from build123d import *

# Parameters (mm, degrees)
BOSS_EXTRUDE1_DEPTH = 25
SKETCH2_R           = 2.6
CUT_EXTRUDE1_DEPTH  = 8
CUT_EXTRUDE2_DEPTH  = 25.75
FILLET1_R           = 4
CHAMFER1_SIZE       = 2
CHAMFER2_SIZE       = 1


with BuildPart() as part:
    # Sketch1 → Boss-Extrude1 (new body)
    with BuildSketch(Plane.XY):
        Polygon((0, 14), (0, -14), (7, -14), (7, -5.5), (15, -5.5), (15, -10.75), (24, -10.75), (24, 10.75), (15, 10.75), (15, 5.5), (7, 5.5), (7, 14), align=None)
    extrude(amount=BOSS_EXTRUDE1_DEPTH)

    # Sketch2 → Cut-Extrude1 (cut)
    with BuildSketch(Plane.ZY):
        with Locations(Location((5, 9, 0), (0, 0, 270))):  # turned: the seam where the file's is
            Circle(SKETCH2_R)
        with Locations(Location((20, 9, 0), (0, 0, 270))):  # turned: the seam where the file's is
            Circle(SKETCH2_R)
        with Locations(Location((5, -8, 0), (0, 0, 270))):  # turned: the seam where the file's is
            Circle(SKETCH2_R)
        with Locations(Location((20, -8, 0), (0, 0, 270))):  # turned: the seam where the file's is
            Circle(SKETCH2_R)
    extrude(amount=-CUT_EXTRUDE1_DEPTH, mode=Mode.SUBTRACT)

    # Sketch3 → Cut-Extrude2 (cut, through all)
    with BuildSketch(Plane(origin=(0, 10.75, 0), x_dir=(1, 0, 0), z_dir=(0, 1, 0))):
        Polygon((24, 0), (23.5, -25), (24, -25), align=None)
    extrude(amount=-CUT_EXTRUDE2_DEPTH, mode=Mode.SUBTRACT)

    # Fillet1
    fillet1_edges = [part.edges().sort_by_distance(p)[0] for p in [
        (3.5, -14, 25),
        (3.5, -14, 0),
        (3.5, 14, 0),
        (3.5, 14, 25),
    ]]
    fillet(fillet1_edges, radius=FILLET1_R)

    # Chamfer1
    chamfer1_edges = [part.edges().sort_by_distance(p)[0] for p in [
        (19.25, -10.75, 25),
        (19.25, 10.75, 25),
    ]]
    chamfer(chamfer1_edges, length=CHAMFER1_SIZE)

    # Chamfer2
    chamfer2_edges = [part.edges().sort_by_distance(p)[0] for p in [
        (15, -10.75, 11.5),
        (15, 10.75, 11.5),
        (23.77, -10.75, 11.5),
        (23.77, 10.75, 11.5),
    ]]
    chamfer(chamfer2_edges, length=CHAMFER2_SIZE)


solid = part.part
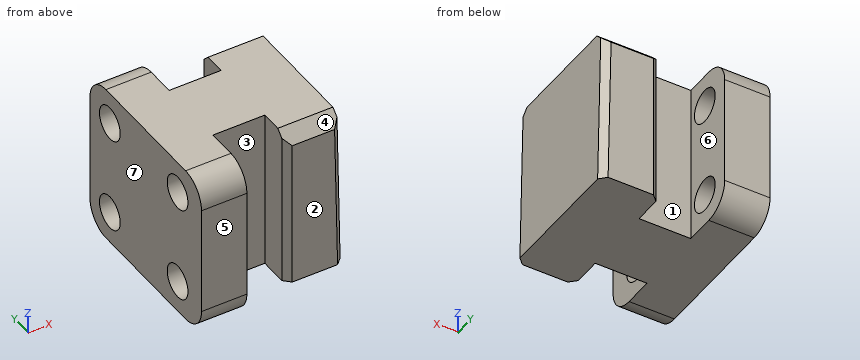
Geometry: final body of the model. Coordinates: model frame, mm. Face numbers are marked on the shaded views. A direction names the side the tool comes from. Coordinates: 2 decimals unless noted, no trailing zeros. Order: outer loops, then holes, each group sorted by start corner. A loop starts at its lowest first (then second) coordinate and runs counter-clockwise, first axis right, second up. Notation, with made-up numbers: (-33.75, -31.75) - (13.25, -31.75) arc R10 cw to (13.25, -13.75) - close; hole circle Ø7 at (86.5, 49). An arc over 180 degrees is marked (long way). Use one line per item in the form item = value.
1) Pin query (flat end, axial travel): pin 1 (7.5 mm diameter, centred on x = 18, z = 8, fed in from -Y); pin 2 (7.5 mm diameter, centred on x = 19, z = 8, fed in from +Y); pin 3 (4 mm diameter, centred on x = 12.5, z = 13, fed in from +Y). Return the tip coordinate at first contact, or that it passes through.
Solutions:
pin_1 = -10.75
pin_2 = 10.75
pin_3 = 5.5
2) Section D-D (x = 2). Return loops of the section in (y, z), then the cut area to 3 significant figures.
Solutions:
outline = (-14, 4) arc R4 ccw to (-10, 0) - (10, 0) arc R4 ccw to (14, 4) - (14, 21) arc R4 ccw to (10, 25) - (-10, 25) arc R4 ccw to (-14, 21) - close; hole circle Ø5.2 at (-8, 5); hole circle Ø5.2 at (-8, 20); hole circle Ø5.2 at (9, 5); hole circle Ø5.2 at (9, 20)
area = 601 mm^2
3) Section B-B (x = 7.5). Return loops of the section in (y, z).
Solutions:
outline = (-5.5, 0) - (5.5, 0) - (5.5, 25) - (-5.5, 25) - (-5.5, 20.71) arc R2.6 cw to (-5.5, 19.29) - (-5.5, 5.71) arc R2.6 cw to (-5.5, 4.29) - close
4) Section C-C (z = 20). Return loops of the section in (x, y), then the cut area to 3 significant figures.
Solutions:
outline = (0, -14) - (7, -14) - (7, -10.6) - (0, -10.6) - close; (0, -5.4) - (8, -5.4) - (8, -5.5) - (15, -5.5) - (15, -9.75) - (16, -10.75) - (22.6, -10.75) - (23.6, -9.75) - (23.6, 9.75) - (22.6, 10.75) - (16, 10.75) - (15, 9.75) - (15, 5.5) - (7, 5.5) - (7, 6.4) - (0, 6.4) - close; (0, 11.6) - (7, 11.6) - (7, 14) - (0, 14) - close
area = 394 mm^2
5) Mould query, pull axis X, two halves, no side actions, for the marked faces 5, 6 and 7. Classes: +X half, -X half, draft (parallel to the pull), parting line (faces both ways), or undercut.
Solutions:
face_5 = draft
face_6 = undercut
face_7 = -X half
6) Ray query, L1, parallel to Z at x = 2.75, y = -8; L2, parallel to Y at x = 5.5, z = 3.25; L3, parallel to Y at x = 16.5, z = 8.75. Return the intervals inside material, ascending.
Solutions:
L1 = 0 to 2.4, 7.6 to 17.4, 22.6 to 25
L2 = -13.93 to -9.92, -6.08 to 7.08, 10.92 to 13.93
L3 = -10.75 to 10.75
7) Section A-A (y = -8). Return loops of the section in (x, z).
Solutions:
outline = (0, 0) - (7, 0) - (7, 2.4) - (0, 2.4) - close; (0, 7.6) - (7, 7.6) - (7, 17.4) - (0, 17.4) - close; (0, 22.6) - (7, 22.6) - (7, 25) - (0, 25) - close; (15, 0) - (24, 0) - (23.5, 25) - (15, 25) - close
8) Set-up query: the marked faces 1, 2, 3 and 4. Return all of +Z, -Z, +X, -X, +Y, -Y with unobstructed straight access to the full face (end or side cutting, diameter ignored); none if empty.
Solutions:
face_1 = +Z, -Z, +Y
face_2 = +Z, -Z, +X, -Y
face_3 = +Z, -Z, -Y
face_4 = +Z, +X, -Y
